Job drawing, mm, ordinate dimensions from the low corner. One solid piece. Give positions to 0.01 mm unless a question says otherwise; leave off trailing zeros. Loops run counter-clockwise (first coordinate to the right, second up) from the corner with the lowest first, then second, coordinate; pieces in that order, holes last. Notation, with made-up numbers: M -1.75,1.5 L 14.25,1.5 A20 ccw 14.25,38.5 Z; hole C -22,-29 d2. An arc over 180 degrees is marked long. One line per question, with ' | ' between items.
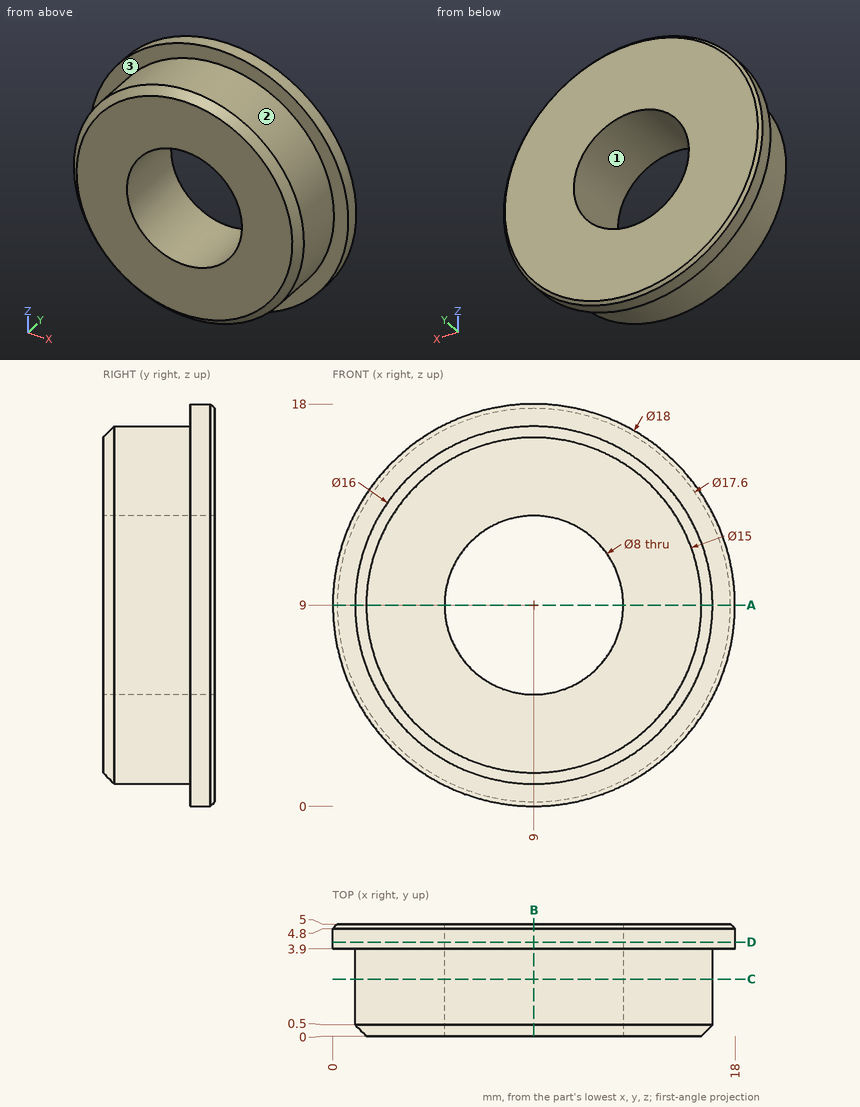
Item 1: Mould opens along Z. For the marked faces 1, 2 and 3 say: pulls with the +Z half, pulls with the -Z half, needs draft (parallel to the pull), parting line crosses it, or undercut.
Conclusion:
face 1: undercut | face 2: parting line crosses it | face 3: needs draft
Item 2: Drill centre lines: line 1 along X through (y, z) = (4, 9); line 2 along X through (y, z) = (3.1, 9); line 3 along Y through (x, z) = (5, 1.5). Where is each one in solid material? Low to high. Write a range as [from, to].
Conclusion:
line 1: [0, 5], [13, 18] | line 2: [1, 5], [13, 17] | line 3: [3.9, 5]
Item 3: Saw through at A-A on z = 9. Give the cut face in (x, y), and give its area (3 significant figures).
Conclusion:
outline: M 0,3.9 L 1,3.9 L 1,0.5 L 1.5,0 L 5,0 L 5,5 L 0.2,5 L 0,4.8 Z; M 13,0 L 16.5,0 L 17,0.5 L 17,3.9 L 18,3.9 L 18,4.8 L 17.8,5 L 13,5 Z | area: 41.9 mm²
Item 4: Drop flat-ended pins along their axis: P1, Ø1.5, axis at y = 1, z = 11.5, coming from the -X side; P2, Ø1, axis at y = 2.5, z = 6, coming from the -X side; P3, Ø1.5, axis at x = 15, y = 1.5, coming from the +Z side. Give the stop position or say it passes through.
Conclusion:
P1: x = 1.19 | P2: x = 1.4 | P3: z = 15.04
Item 5: Saw through at C-C on y = 2.55. Give the cut face in (x, z), and give its area (3 significant figures).
Conclusion:
outline: C 9,9 d16; hole C 9,9 d8 | area: 151 mm²
Item 6: Saw through at D-D on y = 4.2. Give the cut face in (x, z).
Conclusion:
outline: C 9,9 d18; hole C 9,9 d8
Item 7: Saw through at B-B on x = 9. Give the cut face in (y, z).
Conclusion:
outline: M 0,1.5 L 0.5,1 L 3.9,1 L 3.9,0 L 4.8,0 L 5,0.2 L 5,5 L 0,5 Z; M 0,13 L 5,13 L 5,17.8 L 4.8,18 L 3.9,18 L 3.9,17 L 0.5,17 L 0,16.5 Z
